The model under review builds one solid part; all positions refer to its coordinate system, in mm. A direction names the side the tool comes from. Round coordinates to 2 decimals unless told otherwise and drop trailing zeros. Loops run counter-clockwise (first coordinate to the right, second up) from the corner with the lowest first, then second, coordinate; pieces in that order, holes last. Notation, with made-up numbers: M 14.25,-9 L 67.25,-9 A19 ccw 67.25,-4 Z; hole C 42,-14 d2. An arc over 180 degrees is marked long. One line per question, with ' | ' between items.
Autodesk Inventor part; units mm, degrees
ref_plane "YZ Plane" through (0, 0, 0) normal (1, 0, 0) x (0, 1, 0)
ref_plane "XZ Plane" through (0, 0, 0) normal (0, 1, 0) x (-1, 0, 0)
ref_plane "XY Plane" through (0, 0, 0) normal (0, 0, 1) x (1, 0, 0)
sketch "Náčrt1" plane through (0, 0, 0) normal (0, 0, 1) x (1, 0, 0)
  line L0 (0, 8.68) -> (0, -8.68)
  line L1 (-8.68, 0) -> (8.68, 0)
  circle A0 centre (0, 0) radius 6.2
  dimension "d0" = 12.4
extrude "Vysunutí1" add sketch "Náčrt1" along normal blind 1
sketch "Náčrt2" plane through (0, 0, 1) normal (0, 0, 1) x (1, 0, 0)
  line L0 (-8.68, 0) -> (8.68, 0)
  line L1 (0, 8.68) -> (0, -8.68)
  line L2 (-5.5, 0) -> (-5.5, -2.2)
  line L3 (-5.5, -2.2) -> (0, 2.8)
  line L4 (-5.5, 0) -> (0, 5)
  line L5 (5.5, 0) -> (0, 5)
  line L6 (0, 2.8) -> (5.5, -2.2)
  line L7 (5.5, -2.2) -> (5.5, 0)
  point P0 (0, 0)
  dimension "d3" = 2.2
  dimension "d4" = 2.2
  dimension "d5" = 5.5
  dimension "d6" = 5.5
  dimension "d7" = 5
  dimension "d8" = 2.2
extrude "Vysunutí2" add sketch "Náčrt2" along normal blind 0.4 contours L4 L1 L3 L0 | L0 L3 L2 | L5 L0 L6 L1 | L7 L6 L0
properties part number "button_plate_arrow"
1) Add section D-D on x = 1.75. State the section outline as (y, z) points.
Output values:
outline: M -5.95,0 L 5.95,0 L 5.95,1 L 3.41,1 L 3.41,1.4 L 1.21,1.4 L 1.21,1 L -5.95,1 Z
2) Mouldability with a two-part tool opening along X and no side actions: class faces 1 (the flat face through (2.789, 2.465, 1.197)), 2 (the flat face through (0, 3, 1.4)), 3 (the flat face through (0, 0, 1)) as +X half, -X half, draft (parallel to the pull), parting line (faces both ways), or undercut.
Output values:
face 1: +X half | face 2: draft | face 3: undercut
3) For line 1 (Z direction, x = -3.5, y = -2.5); line 2 (X direction, y = -3, z = 0.5); line 3 (Y direction, x = -3.75, z = 0.3), list the stretches that pass through material, from the lowest coordinate up.
Output values:
line 1: z = 0 to 1 | line 2: x = -5.43 to 5.43 | line 3: y = -4.94 to 4.94
4) Add section C-C on z = 0.55. State the section outline as (x, y) points.
Output values:
outline: C 0,0 d12.4
5) Add section B-B on x = 3. State the section outline as (y, z) points.
Output values:
outline: M -5.43,0 L 5.43,0 L 5.43,1 L 2.27,1 L 2.27,1.4 L 0.07,1.4 L 0.07,1 L -5.43,1 Z
6) Add section A-A on y = 1.5. State the section outline as (x, z) points.
Output values:
outline: M -6.02,0 L 6.02,0 L 6.02,1 L 3.85,1 L 3.85,1.4 L 1.43,1.4 L 1.43,1 L -1.43,1 L -1.43,1.4 L -3.85,1.4 L -3.85,1 L -6.02,1 Z
7) Machinability: for faces 4 (the flat face through (-2.789, 2.465, 1.197)), 5 (the flat face through (0, 0, 0)), 6 (the flat face through (2.712, 0.335, 1.197)), which of the approach directions +Z, -Z, +X, -X, +Y, -Y give a long, thin tool a straight path to every point of the face, cutting with its end or side? Answer none if there is none.
Output values:
face 4: +Z, -X, +Y | face 5: -Z, +X, -X, +Y, -Y | face 6: +Z, -Y
